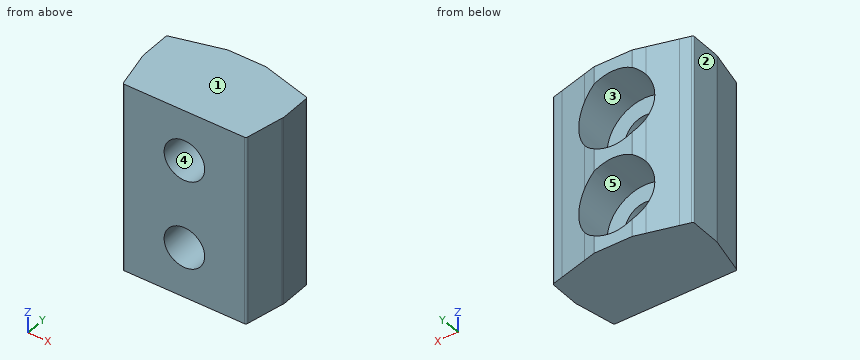
```python
from build123d import *

# Parameters (mm, degrees)
BOSS_EXTRUDE1_DEPTH = 30
SKETCH2_R           = 3.2
CUT_EXTRUDE3_DEPTH  = 37.096941552
SKETCH4_R           = 6
CUT_EXTRUDE4_DEPTH  = 7


with BuildPart() as part:
    # Sketch1 → Boss-Extrude1 (new body)
    with BuildSketch(Plane.XY):
        with BuildLine():
            Line((-5.607917396, 9.03308876), (-1.173065904, 10.221403636))
            Line((-1.173065904, 10.221403636), (0.621358385, 10.702218175))
            ThreePointArc((0.621358385, 10.702218175), (0.659846241, 10.709873886), (0.699004099, 10.712440427))
            Line((0.699004099, 10.712440427), (6.6200126, 10.712440427))
            ThreePointArc((6.6200126, 10.712440427), (6.659170458, 10.709873886), (6.697658314, 10.702218175))
            Line((6.697658314, 10.702218175), (8.492082604, 10.221403636))
            Line((8.492082604, 10.221403636), (12.926934096, 9.03308876))
            Line((12.926934096, 9.03308876), (14.537154063, 8.60163162))
            ThreePointArc((14.537154063, 8.60163162), (14.697514352, 8.494482301), (14.75950835, 8.311853872))
            Line((14.75950835, 8.311853872), (14.75950835, 3.414909596))
            ThreePointArc((14.75950835, 3.414909596), (14.752913122, 3.352350508), (14.73341742, 3.29254203))
            Line((14.73341742, 3.29254203), (14.669480377, 3.149424564))
            Line((14.669480377, 3.149424564), (13.439893107, -2.594399862))
            ThreePointArc((13.439893107, -2.594399862), (13.352025142, -2.806531896), (13.139893107, -2.894399862))
            Line((13.139893107, -2.894399862), (-5.820876408, -2.894399862))
            ThreePointArc((-5.820876408, -2.894399862), (-6.033008442, -2.806531896), (-6.120876408, -2.594399862))
            Line((-6.120876408, -2.594399862), (-7.41440072, 3.29254203))
            ThreePointArc((-7.41440072, 3.29254203), (-7.433896423, 3.352350508), (-7.44049165, 3.414909596))
            Line((-7.44049165, 3.414909596), (-7.44049165, 8.311853872))
            ThreePointArc((-7.44049165, 8.311853872), (-7.378497652, 8.494482301), (-7.218137364, 8.60163162))
            Line((-7.218137364, 8.60163162), (-5.607917396, 9.03308876))
        make_face()
    extrude(amount=BOSS_EXTRUDE1_DEPTH)

    # Sketch2 → Cut-Extrude3 (cut, through all)
    with BuildSketch(Plane.XZ.offset(2.894399862)):
        with Locations((3.65950835, 22)):
            Circle(SKETCH2_R)
        with Locations((3.65950835, 8)):
            Circle(SKETCH2_R)
    extrude(amount=-CUT_EXTRUDE3_DEPTH, mode=Mode.SUBTRACT)

    # Sketch4 → Cut-Extrude4 (cut)
    with BuildSketch(Plane(origin=(0, 10.712440427, 0), x_dir=(1, 0, 0), z_dir=(0, 1, 0))):
        with Locations(Location((3.65950835, -8, 0), (0, 0, 270))):
            Circle(SKETCH4_R)
        with Locations(Location((3.65950835, -22, 0), (0, 0, 270))):
            Circle(SKETCH4_R)
    extrude(amount=-CUT_EXTRUDE4_DEPTH, mode=Mode.SUBTRACT)


solid = part.part
```
Can you work these out from the model? Positions are in its coordinate system, mm. Face numbers are marked on the shaded views. A direction names the side the tool comes from. Give positions to 0.01 mm unless a question says otherwise; leave off trailing zeros. Write each loop counter-clockwise with the first axis right and the second up, starting at its lowest first coordinate (ties: lowest second). Pieces come first, ordered by that corner, then holes. Notation, with made-up numbers: (15.25, 82.25) -> (51.25, 82.25) arc R25 cw to (51.25, 120.25) -> close; hole circle Ø11 at (75.5, 60.5). An arc over 180 degrees is marked (long way). Write item = value, one per line.
(1) I'm going to push flat-ended pins straight in: P1, Ø3.5, axis at x = 2, z = 24.5, coming from the +Y side; P2, Ø5, axis at x = 3.66, z = 22, coming from the +Y side; P3, Ø1.5, axis at y = -1.5, z = 18, coming from the -X side. Where does each tip first touch, or does it pass through?
Worked out:
P1 = 3.71
P2 = through
P3 = -6.53
(2) Thinking about a two-plate mould opening in Z: for the marked faces 1, 2 and 3, which applies, released by +Z, released by -Z, zero draft, split by the parting line, or undercut?
Worked out:
face_1 = released by +Z
face_2 = zero draft
face_3 = undercut
(3) For the marked faces 4 and 5, which set-ups out of +Z, -Z, +X, -X, +Y, -Y let a thin tool reach every point of the face, with its end or its side?
Worked out:
face_4 = +Y, -Y
face_5 = +Y
(4) Suppose I cut it at A-A on x = 5.5. Write out the boundary of the cut face in (y, z), then the cut area to 3 significant figures.
Worked out:
outline = (-2.89, 0) -> (10.71, 0) -> (10.71, 2.29) -> (3.71, 2.29) -> (3.71, 5.38) -> (-2.89, 5.38) -> close; (-2.89, 10.62) -> (3.71, 10.62) -> (3.71, 13.71) -> (10.71, 13.71) -> (10.71, 16.29) -> (3.71, 16.29) -> (3.71, 19.38) -> (-2.89, 19.38) -> close; (-2.89, 24.62) -> (3.71, 24.62) -> (3.71, 27.71) -> (10.71, 27.71) -> (10.71, 30) -> (-2.89, 30) -> close
area = 179 mm^2
(5) Suppose I cut it at D-D on z = 8. Write out the boundary of the cut face in (x, y), then the cut area to 3 significant figures.
Worked out:
outline = (-7.44, 3.41) arc R0.3 ccw to (-7.41, 3.29) -> (-6.12, -2.59) arc R0.3 ccw to (-5.82, -2.89) -> (0.46, -2.89) -> (0.46, 3.71) -> (-2.34, 3.71) -> (-2.34, 9.91) -> (-7.22, 8.6) arc R0.3 ccw to (-7.44, 8.31) -> close; (6.86, -2.89) -> (13.14, -2.89) arc R0.3 ccw to (13.44, -2.59) -> (14.67, 3.15) -> (14.73, 3.29) arc R0.3 ccw to (14.76, 3.41) -> (14.76, 8.31) arc R0.3 ccw to (14.54, 8.6) -> (9.66, 9.91) -> (9.66, 3.71) -> (6.86, 3.71) -> close
area = 152 mm^2
(6) I need wall thicknesses on probe 1 along Z at (x, y) = (5, 1.5); probe 2 along Z at (x, y) = (6.75, 9.5); probe 3 along X at (y, z) = (8.5, 22). Which ranges of each line are inside material? Lowest first, please. Write a range as from..to.
Worked out:
probe_1 = 0..5.09, 10.91..19.09, 24.91..30
probe_2 = 0..2.86, 13.14..16.86, 27.14..30
probe_3 = -7.37..-2.34, 9.66..14.69
(7) Suppose I cut it at B-B on z = 23. Write out the boundary of the cut face in (x, y).
Worked out:
outline = (-7.44, 3.41) arc R0.3 ccw to (-7.41, 3.29) -> (-6.12, -2.59) arc R0.3 ccw to (-5.82, -2.89) -> (0.62, -2.89) -> (0.62, 3.71) -> (-2.26, 3.71) -> (-2.26, 9.93) -> (-7.22, 8.6) arc R0.3 ccw to (-7.44, 8.31) -> close; (6.7, -2.89) -> (13.14, -2.89) arc R0.3 ccw to (13.44, -2.59) -> (14.67, 3.15) -> (14.73, 3.29) arc R0.3 ccw to (14.76, 3.41) -> (14.76, 8.31) arc R0.3 ccw to (14.54, 8.6) -> (9.58, 9.93) -> (9.58, 3.71) -> (6.7, 3.71) -> close
(8) Suppose I cut it at C-C on y = 2. Write out the boundary of the cut face in (x, z).
Worked out:
outline = (-7.13, 0) -> (14.42, 0) -> (14.42, 30) -> (-7.13, 30) -> close; hole circle Ø6.4 at (3.66, 8); hole circle Ø6.4 at (3.66, 22)
